from build123d import *

# Parameters (mm, degrees)
SKETCH1_R           = 15
SKETCH1_R_2         = 12.75
BOSS_EXTRUDE1_DEPTH = 17
SKETCH2_R           = 15
BOSS_EXTRUDE2_DEPTH = 0.25


with BuildPart() as part:
    # Sketch1 → Boss-Extrude1 (new body)
    with BuildSketch(Plane.XY):
        Circle(SKETCH1_R)
        Circle(SKETCH1_R_2, mode=Mode.SUBTRACT)
    extrude(amount=BOSS_EXTRUDE1_DEPTH)

    # Sketch2 → Boss-Extrude2 (add)
    with BuildSketch(Plane.XY):
        Circle(SKETCH2_R)
        with BuildLine():
            Line((-0.5, 4.974937186), (-0.5, 8.860904299))
            Line((-0.5, 8.860904299), (-1, 8.860904299))
            Line((-1, 8.860904299), (-1, 7.306888873))
            ThreePointArc((-1, 7.306888873), (-7.375, 0), (-1, -7.306888873))
            Line((-1, -7.306888873), (-1, -8.860904299))
            Line((-1, -8.860904299), (-0.5, -8.860904299))
            Line((-0.5, -8.860904299), (-0.5, -4.974937186))
            ThreePointArc((-0.5, -4.974937186), (-5, 0), (-0.5, 4.974937186))
        make_face(mode=Mode.SUBTRACT)
        with BuildLine():
            Line((1, 7.306888873), (1, 8.860904299))
            Line((1, 8.860904299), (0.5, 8.860904299))
            Line((0.5, 8.860904299), (0.5, 4.974937186))
            ThreePointArc((0.5, 4.974937186), (5, 0), (0.5, -4.974937186))
            Line((0.5, -4.974937186), (0.5, -8.860904299))
            Line((0.5, -8.860904299), (1, -8.860904299))
            Line((1, -8.860904299), (1, -7.306888873))
            ThreePointArc((1, -7.306888873), (7.375, 0), (1, 7.306888873))
        make_face(mode=Mode.SUBTRACT)
        with BuildLine():
            Line((-12.740192306, 0.5), (-8.860904299, 0.5))
            Line((-8.860904299, 0.5), (-8.860904299, 1))
            Line((-8.860904299, 1), (-10.326694776, 1))
            ThreePointArc((-10.326694776, 1), (0, 10.375), (10.326694776, 1))
            Line((10.326694776, 1), (8.860904299, 1))
            Line((8.860904299, 1), (8.860904299, 0.5))
            Line((8.860904299, 0.5), (12.740192306, 0.5))
            ThreePointArc((12.740192306, 0.5), (0, 12.75), (-12.740192306, 0.5))
        make_face(mode=Mode.SUBTRACT)
        with BuildLine():
            Line((-12.740192306, -0.5), (-8.860904299, -0.5))
            Line((-8.860904299, -0.5), (-8.860904299, -1))
            Line((-8.860904299, -1), (-10.326694776, -1))
            ThreePointArc((-10.326694776, -1), (0, -10.375), (10.326694776, -1))
            Line((10.326694776, -1), (8.860904299, -1))
            Line((8.860904299, -1), (8.860904299, -0.5))
            Line((8.860904299, -0.5), (12.740192306, -0.5))
            ThreePointArc((12.740192306, -0.5), (0, -12.75), (-12.740192306, -0.5))
        make_face(mode=Mode.SUBTRACT)
    extrude(amount=-BOSS_EXTRUDE2_DEPTH)


solid = part.part
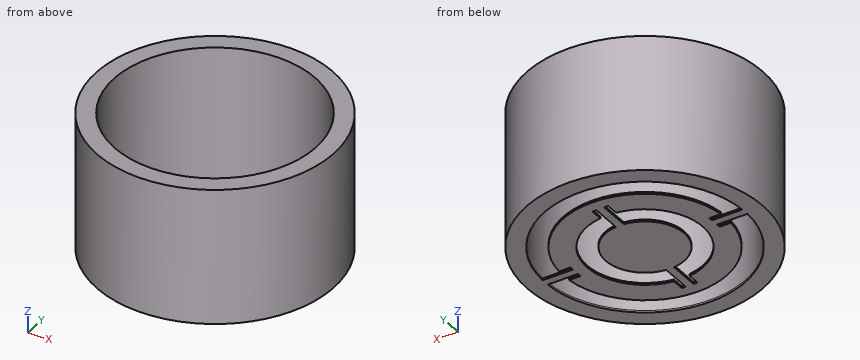
Design review of the part built by this model. Coordinates are the model's own, in mm. Give positions to 0.01 mm unless a question says otherwise; leave off trailing zeros. Order: outer loops, then holes, each group sorted by start corner. A loop starts at its lowest first (then second) coordinate and runs counter-clockwise, first axis right, second up.
1. Add section C-C, the plane y = -6. State the section outline as (x, z) points, then the cut area to 3 significant figures.
Solution:
outline: (-13.75, -0.25) - (-11.25, -0.25) - (-11.25, 17) - (-13.75, 17) - close; (-8.46, -0.25) - (-4.29, -0.25) - (-4.29, 0) - (-8.46, 0) - close; (-0.5, -0.25) - (0.5, -0.25) - (0.5, 0) - (-0.5, 0) - close; (4.29, -0.25) - (8.46, -0.25) - (8.46, 0) - (4.29, 0) - close; (11.25, -0.25) - (13.75, -0.25) - (13.75, 17) - (11.25, 17) - close
area: 88.5 mm2
2. Add section D-D, the plane x = 9.5. State the section outline as (y, z) points, then the cut area to 3 significant figures.
Solution:
outline: (-11.61, -0.25) - (-8.5, -0.25) - (-8.5, 17) - (-11.61, 17) - close; (-4.17, -0.25) - (-1, -0.25) - (-1, 0) - (-4.17, 0) - close; (-0.5, -0.25) - (0.5, -0.25) - (0.5, 0) - (-0.5, 0) - close; (1, -0.25) - (4.17, -0.25) - (4.17, 0) - (1, 0) - close; (8.5, -0.25) - (11.61, -0.25) - (11.61, 17) - (8.5, 17) - close
area: 109 mm2
3. Add section A-A, the plane x = 0. State the section outline as (y, z) points (3 decimals), then the cut area to 3 significant figures.
Solution:
outline: (-15, -0.25) - (-12.75, -0.25) - (-12.75, 17) - (-15, 17) - close; (-10.375, -0.25) - (10.375, -0.25) - (10.375, 0) - (-10.375, 0) - close; (12.75, -0.25) - (15, -0.25) - (15, 17) - (12.75, 17) - close
area: 82.8 mm2
4. Add section B-B, the plane y = 0. State the section outline as (x, z) points (3 decimals), then the cut area to 3 significant figures.
Solution:
outline: (-15, -0.25) - (-7.375, -0.25) - (-7.375, 0) - (-12.75, 0) - (-12.75, 17) - (-15, 17) - close; (-5, -0.25) - (5, -0.25) - (5, 0) - (-5, 0) - close; (7.375, -0.25) - (15, -0.25) - (15, 17) - (12.75, 17) - (12.75, 0) - (7.375, 0) - close
area: 82.8 mm2
5. For pin 1 Ø1 at (x, y) = (5, -1.5) entering from -Z; pin 2 Ø2 at (x, z) = (11.5, 13) entering from +Y; pin 3 Ø4 at (y, z) = (-11.5, 8) entering from -X; pin 4 Ø4 at (x, z) = (9.5, 13) entering from -Y, all flat-tipped, find the tip position at first contact; note any pin that passes through.
Solution:
pin 1: stops at z = -0.25
pin 2: stops at y = 10.71
pin 3: stops at x = -11.61
pin 4: stops at y = -12.99
6. To check wall thickness, follow L1, parallel to Y at x = 0, z = 10.5; L2, parallel to Y at x = 4.5, z = 6.25. State the ranges of each line that lie inside material, in increasing order.
Solution:
L1: y = -15 to -12.75, 12.75 to 15
L2: y = -14.31 to -11.93, 11.93 to 14.31
